```python
from build123d import *

# Parameters (mm, degrees)
SKETCH_1_R               = 7.5
EXTRUDE_1_DEPTH          = 2.5
SKETCH_2_R               = 5
EXTRUDE_2_DEPTH          = 1
SKETCH_3_R               = 2.45
EXTRUDE_3_DEPTH          = 18
SKETCH_4_R               = 1
CUT_EXTRUDE_1_DEPTH      = 10
CUT_EXTRUDE_2_DEPTH      = 3.1
CUT_EXTRUDE_2_DEPTH_BACK = 3.1
SKETCH_5_R               = 3


with BuildPart() as part:
    # 스케치1 → 보스-돌출1 (new body)
    with BuildSketch(Plane.XY):
        Circle(SKETCH_1_R)
    extrude(amount=EXTRUDE_1_DEPTH)

    # 스케치2 → 보스-돌출2 (add)
    with BuildSketch(Plane.XY.offset(2.5)):
        Circle(SKETCH_2_R)
    extrude(amount=EXTRUDE_2_DEPTH)

    # 스케치3 → 보스-돌출3 (add)
    with BuildSketch(Plane.XY.offset(3.5)):
        Circle(SKETCH_3_R)
    extrude(amount=EXTRUDE_3_DEPTH)

    # 스케치4 → 컷-돌출1 (cut)
    with BuildSketch(Plane.XY.offset(21.5)):
        Circle(SKETCH_4_R)
    extrude(amount=-CUT_EXTRUDE_1_DEPTH, mode=Mode.SUBTRACT)

    # 스케치5 → 컷-돌출2 (cut, two sides: drawn at the far end of the back side and taken through both)
    with BuildSketch(Plane(origin=(0, 0, 0), x_dir=(1, 0, 0), z_dir=(0, 1, 0)).offset(-CUT_EXTRUDE_2_DEPTH_BACK)):
        Circle(SKETCH_5_R)
    extrude(amount=CUT_EXTRUDE_2_DEPTH + CUT_EXTRUDE_2_DEPTH_BACK, mode=Mode.SUBTRACT)


solid = part.part
```
Geometry check sheet. Reference: the model listing, model coordinates, mm. A direction names the side the tool comes from. Coordinates: 2 decimals unless noted, no trailing zeros. Order: outer loops, then holes, each group sorted by start corner. A loop starts at its lowest first (then second) coordinate and runs counter-clockwise, first axis right, second up.
Item 1: Section check D-D (y = 3.75). Enter the section's corners in (x, z).
Item 2: Section check B-B (y = 0). Enter the section's corners in (x, z).
Item 3: Mould release check, pull along Y, two halves, no side actions. Record for faces 1 (the flat face through (2, -5, 2.5)), 2 (the flat face through (0, 0, 11.5)), 3 (the cylindrical face through (-7.493, 0.33, 1.232)): released by +Y, released by -Y, zero draft, split by the parting line, or undercut.
Item 4: Scan lines: line 1 along Y through (x, z) = (0, 14.5); line 2 along X through (y, z) = (0.5, 14.75); line 3 along Z through (x, y) = (5.75, 1.25). Record each from-to range of solid material in increasing order.
Item 5: Section check C-C (z = 16.5). Enter the section's corners in (x, y).
Item 6: Depth check by flat-ended pin: pin 1 (1.5 mm diameter, centred on x = 1, z = 1.5, fed in from +Y); pin 2 (1.5 mm diameter, centred on x = -3, z = 5, fed in from +Y); pin 3 (6 mm diameter, centred on y = 3, z = 16.5, fed in from +X); pin 4 (3 mm diameter, centred on x = 4, z = 9.5, fed in from -Y). Enter the tip coordinate at first touch or a pass-through.
Item 7: Section check A-A (x = 0). Enter the section's corners in (y, z).
Item 8: Tool access check on faces 4 (the cylindrical face through (-1.08, -4.88, 2.99)), 5 (the flat face through (1, -1, 21.5)), 6 (the flat face through (0, -3.1, 1)). Record the directions out of +Z, -Z, +X, -X, +Y, -Y that give a thin tool (end or side, any length) a straight path to the whole face; none if there is none.
Check sheet entries:
1. outline: (-6.5, 0) - (6.5, 0) - (6.5, 2.5) - (3.31, 2.5) - (3.31, 3.5) - (-3.31, 3.5) - (-3.31, 2.5) - (-6.5, 2.5) - close
2. outline: (-7.5, 0) - (-3, 0) arc R3 cw to (3, 0) - (7.5, 0) - (7.5, 2.5) - (5, 2.5) - (5, 3.5) - (2.45, 3.5) - (2.45, 21.5) - (1, 21.5) - (1, 11.5) - (-1, 11.5) - (-1, 21.5) - (-2.45, 21.5) - (-2.45, 3.5) - (-5, 3.5) - (-5, 2.5) - (-7.5, 2.5) - close
3. face 1: zero draft
3. face 2: undercut
3. face 3: split by the parting line
4. line 1: y = -2.45 to -1, 1 to 2.45
4. line 2: x = -2.4 to -0.87, 0.87 to 2.4
4. line 3: z = 0 to 2.5
5. outline: circle Ø4.9 at (0, 0); hole circle Ø2 at (0, 0)
6. pin 1: stops at y = 7.5
6. pin 2: stops at y = 0.97
6. pin 3: stops at x = 2.45
6. pin 4: passes through
7. outline: (-7.5, 0) - (-3.1, 0) - (-3.1, 3) - (3.1, 3) - (3.1, 0) - (7.5, 0) - (7.5, 2.5) - (5, 2.5) - (5, 3.5) - (2.45, 3.5) - (2.45, 21.5) - (1, 21.5) - (1, 11.5) - (-1, 11.5) - (-1, 21.5) - (-2.45, 21.5) - (-2.45, 3.5) - (-5, 3.5) - (-5, 2.5) - (-7.5, 2.5) - close
8. face 4: +Z
8. face 5: +Z, +X, -X, +Y, -Y
8. face 6: -Z
